```python
from build123d import *

# Parameters (mm, degrees)
F0_W     = 12.75
F0_H     = 6
F1_DEPTH = 21.9
F2_R     = 2.99999
F3_R     = 1.5
F4_DEPTH = 10
F6_DEPTH = 1.3


# Not quite as in the source:
# - a fillet or chamfer is up to 0.001 mm smaller than in the source, because OpenCascade refuses the exact size


with BuildPart() as f1:
    # F0 (on Top) → F1 (new body)
    with BuildSketch(Plane.XY):
        Rectangle(F0_W, F0_H)
    extrude(amount=F1_DEPTH)

    # F2 (radius 3 in the source; OpenCascade refuses exactly that, so slightly less here)
    f2_edges = [f1.edges().sort_by_distance(p)[0] for p in [
        (-6.375, -3, 10.95),
        (-6.375, 3, 10.95),
        (6.375, -3, 10.95),
        (6.375, 3, 10.95),
    ]]
    fillet(f2_edges, radius=F2_R)

    # F3 (on face) → F4 (join)
    with BuildSketch(Plane(origin=(0, 0, 0), x_dir=(1, 0, 0), z_dir=(0, 0, -1))):
        Circle(F3_R)
    extrude(amount=F4_DEPTH)

    # F5 (on face) → F6 (cut)
    with BuildSketch(Plane.XY.offset(21.9)):
        with BuildLine():
            Line((3.375, 2.35), (-3.375, 2.35))
            ThreePointArc((-3.375, 2.35), (-5.725, 0), (-3.375, -2.35))
            Line((-3.375, -2.35), (3.375, -2.35))
            ThreePointArc((3.375, -2.35), (5.725, 0), (3.375, 2.35))
        make_face()
    extrude(amount=-F6_DEPTH, mode=Mode.SUBTRACT)


solid = f1.part
```
Geometry check sheet. Reference: the model listing, model coordinates, mm. A direction names the side the tool comes from. Coordinates: 2 decimals unless noted, no trailing zeros. Write each loop counter-clockwise with the first axis right and the second up, starting at its lowest first coordinate (ties: lowest second). Pieces come first, ordered by that corner, then holes. Notation, with made-up numbers: M -30,-39 L -8,-39 A24 ccw -8,-24 Z; hole C -16,2 d2. An arc over 180 degrees is marked long. Answer as a JSON object with one key per item and string values.
1. Scan lines: L1, parallel to Z at x = 3, y = 2.75; L2, parallel to Z at x = 0.5, y = -0.5; L3, parallel to Y at x = -4, z = 19. Record each from-to range of solid material in increasing order.
Answers below:
{"L1": "z = 0 to 21.9", "L2": "z = -10 to 20.6", "L3": "y = -2.93 to 2.93"}
2. Section check D-D, the plane x = 2.25. Enter the section's corners in (y, z).
Answers below:
{"outline": "M -3,0 L 3,0 L 3,21.9 L 2.35,21.9 L 2.35,20.6 L -2.35,20.6 L -2.35,21.9 L -3,21.9 Z"}
3. Section check C-C, the plane y = 0.75. Enter the section's corners in (x, z), plus the area to 3 significant figures.
Answers below:
{"outline": "M -6.28,0 L -1.3,0 L -1.3,-10 L 1.3,-10 L 1.3,0 L 6.28,0 L 6.28,21.9 L 5.6,21.9 L 5.6,20.6 L -5.6,20.6 L -5.6,21.9 L -6.28,21.9 Z", "area": "286 mm²"}
4. Tool access check on faces 4 (the flat face through (0, 0, -10)), 5 (the cylindrical face through (5.724, -0.052, 21.259)). Record the directions out of +Z, -Z, +X, -X, +Y, -Y that give a thin tool (end or side, any length) a straight path to the whole face; none if there is none.
Answers below:
{"face 4": "-Z, +X, -X, +Y, -Y", "face 5": "+Z"}
5. Draft check along Y on faces 1 (the cylindrical face through (-1.5, -0.07, -4.93)), 2 (the flat face through (0, 0, 20.6)), 3 (the flat face through (0, 3, 11)). Enter one of: released by +Y, released by -Y, zero draft, split by the parting line, or undercut.
Answers below:
{"face 1": "split by the parting line", "face 2": "undercut", "face 3": "released by +Y"}
6. Section check A-A, the plane x = 0. Enter the section's corners in (y, z).
Answers below:
{"outline": "M -3,0 L -1.5,0 L -1.5,-10 L 1.5,-10 L 1.5,0 L 3,0 L 3,21.9 L 2.35,21.9 L 2.35,20.6 L -2.35,20.6 L -2.35,21.9 L -3,21.9 Z"}
